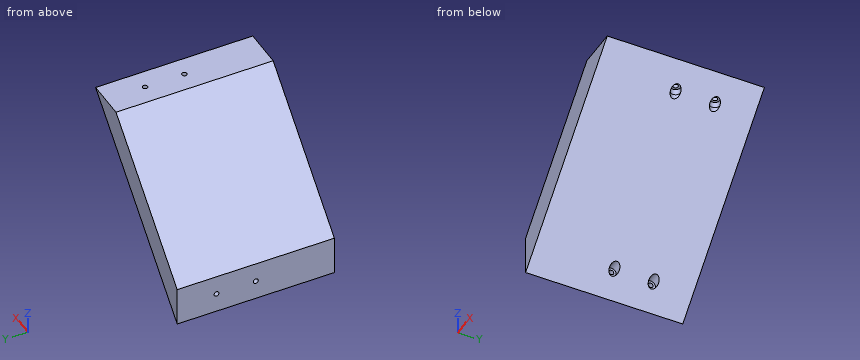
Autodesk Inventor part; units mm, degrees
ref_plane "YZ Plane" through (0, 0, 0) normal (1, 0, 0) x (0, 1, 0)
ref_plane "XZ Plane" through (0, 0, 0) normal (0, 1, 0) x (-1, 0, 0)
ref_plane "XY Plane" through (0, 0, 0) normal (0, 0, 1) x (1, 0, 0)
sketch "Sketch1" plane through (0, 0, 0) normal (0, 1, 0) x (-1, 0, 0)
  line L0 (6.35, 0) -> (1365.25, 0)
  line L1 (1371.6, -6.35) -> (1371.6, -1365.25)
  line L2 (1365.25, -1371.6) -> (6.35, -1371.6)
  line L3 (0, -1365.25) -> (0, -6.35)
  line L4 (1346.2, -1346.2) -> (1346.2, -25.4)
  line L5 (1346.2, -25.4) -> (25.4, -25.4)
  line L6 (25.4, -25.4) -> (25.4, -1346.2)
  line L7 (25.4, -1346.2) -> (1346.2, -1346.2)
  line L8 (1320.8, -50.8) -> (1320.8, -1320.8)
  line L9 (1320.8, -1320.8) -> (50.8, -1320.8)
  line L10 (50.8, -1320.8) -> (50.8, -50.8)
  line L11 (50.8, -50.8) -> (1320.8, -50.8)
  line L12 (1320.8, -50.8) -> (1346.2, -25.4)
  line L13 (1320.8, -1320.8) -> (1346.2, -1346.2)
  line L14 (50.8, -1320.8) -> (25.4, -1346.2)
  line L15 (50.8, -50.8) -> (25.4, -25.4)
  line L16 (1219.2, -482.6) -> (1016, -482.6)
  line L17 (1016, -482.6) -> (1016, -889)
  line L18 (1016, -889) -> (1219.2, -889)
  line L19 (1219.2, -889) -> (1219.2, -482.6)
  line L20 (355.6, -482.6) -> (152.4, -482.6)
  line L21 (152.4, -482.6) -> (152.4, -889)
  line L22 (152.4, -889) -> (355.6, -889)
  line L23 (355.6, -889) -> (355.6, -482.6)
  line L24 (889, -1016) -> (482.6, -1016)
  line L25 (482.6, -1016) -> (482.6, -1219.2)
  line L26 (482.6, -1219.2) -> (889, -1219.2)
  line L27 (889, -1219.2) -> (889, -1016)
  line L28 (889, -152.4) -> (482.6, -152.4)
  line L29 (482.6, -152.4) -> (482.6, -355.6)
  line L30 (482.6, -355.6) -> (889, -355.6)
  line L31 (889, -355.6) -> (889, -152.4)
  circle A0 centre (685.8, -685.8) radius 254
  line L32 (889, -127) -> (482.6, -127)
  line L33 (457.2, -127) -> (457.2, -381)
  line L34 (457.2, -381) -> (914.4, -381)
  line L35 (914.4, -381) -> (914.4, -127)
  line L36 (1244.6, -457.2) -> (990.6, -457.2)
  line L37 (990.6, -457.2) -> (990.6, -914.4)
  line L38 (990.6, -914.4) -> (1244.6, -914.4)
  line L39 (1244.6, -889) -> (1244.6, -482.6)
  line L40 (914.4, -990.6) -> (457.2, -990.6)
  line L41 (457.2, -990.6) -> (457.2, -1244.6)
  line L42 (482.6, -1244.6) -> (889, -1244.6)
  line L43 (914.4, -1244.6) -> (914.4, -990.6)
  line L44 (381, -457.2) -> (127, -457.2)
  line L45 (127, -482.6) -> (127, -889)
  line L46 (127, -914.4) -> (381, -914.4)
  line L47 (381, -914.4) -> (381, -457.2)
  line L48 (152.4, -482.6) -> (50.8, -482.6)
  line L49 (127, -457.2) -> (50.8, -457.2)
  line L50 (152.4, -889) -> (50.8, -889)
  line L51 (127, -914.4) -> (50.8, -914.4)
  line L52 (355.6, -889) -> (381, -889)
  line L53 (355.6, -482.6) -> (381, -482.6)
  line L54 (457.2, -1244.6) -> (457.2, -1320.8)
  line L55 (482.6, -1219.2) -> (482.6, -1320.8)
  line L56 (889, -1219.2) -> (889, -1320.8)
  line L57 (914.4, -1244.6) -> (914.4, -1320.8)
  line L58 (1244.6, -914.4) -> (1320.8, -914.4)
  line L59 (1219.2, -889) -> (1320.8, -889)
  line L60 (1219.2, -482.6) -> (1320.8, -482.6)
  line L61 (1244.6, -457.2) -> (1320.8, -457.2)
  line L62 (889, -152.4) -> (889, -50.8)
  line L63 (914.4, -127) -> (914.4, -50.8)
  line L64 (482.6, -152.4) -> (482.6, -50.8)
  line L65 (457.2, -127) -> (457.2, -50.8)
  line L66 (889, -1016) -> (889, -990.6)
  line L67 (482.6, -1016) -> (482.6, -990.6)
  line L68 (1016, -889) -> (990.6, -889)
  line L69 (1016, -482.6) -> (990.6, -482.6)
  line L70 (889, -355.6) -> (889, -381)
  line L71 (482.6, -355.6) -> (482.6, -381)
  line L72 (914.4, -381) -> (990.6, -457.2)
  line L73 (990.6, -482.6) -> (889, -381)
  line L74 (990.6, -914.4) -> (914.4, -990.6)
  line L75 (889, -990.6) -> (990.6, -889)
  line L76 (381, -914.4) -> (457.2, -990.6)
  line L77 (482.6, -990.6) -> (381, -889)
  line L78 (457.2, -381) -> (381, -457.2)
  line L79 (482.6, -381) -> (381, -482.6)
  line L80 (1257.3, -50.8) -> (1320.8, -114.3)
  line L81 (1320.8, -1257.3) -> (1257.3, -1320.8)
  line L82 (50.8, -1257.3) -> (114.3, -1320.8)
  line L83 (50.8, -114.3) -> (114.3, -50.8)
  line L84 (68.7605, -132.2605) -> (132.2605, -68.7605)
  line L85 (68.7605, -1239.3395) -> (132.2605, -1302.8395)
  line L86 (1302.8395, -1239.3395) -> (1239.3395, -1302.8395)
  line L87 (1239.3395, -68.7605) -> (1302.8395, -132.2605)
  line L88 (1302.8395, -132.2605) -> (1320.8, -150.221)
  line L89 (1239.3395, -68.7605) -> (1221.379, -50.8)
  line L90 (1302.8395, -1239.3395) -> (1320.8, -1221.379)
  line L91 (1239.3395, -1302.8395) -> (1221.379, -1320.8)
  line L92 (132.2605, -1302.8395) -> (150.221, -1320.8)
  line L93 (68.7605, -1239.3395) -> (50.8, -1221.379)
  line L94 (132.2605, -68.7605) -> (150.221, -50.8)
  line L95 (68.7605, -132.2605) -> (50.8, -150.221)
  line L96 (1365.25, 0) -> (1371.6, -6.35)
  line L97 (1371.6, -1365.25) -> (1365.25, -1371.6)
  line L98 (6.35, -1371.6) -> (0, -1365.25)
  line L99 (6.35, 0) -> (0, -6.35)
  point P0 (0, 0)
  point P1 (1371.6, -1371.6)
  point P2 (1371.6, 0)
  point P3 (0, -1371.6)
  dimension "d0" = 1371.6
  dimension "d1" = 1371.6
  dimension "d2" = 25.4
  dimension "d3" = 25.4
  dimension "d4" = 203.2
  dimension "d5" = 406.4
  dimension "d6" = 203.2
  dimension "d7" = 406.4
  dimension "d8" = 406.4
  dimension "d9" = 203.2
  dimension "d10" = 406.4
  dimension "d11" = 203.2
  dimension "d12" = 101.6
  dimension "d13" = 101.6
  dimension "d14" = 101.6
  dimension "d15" = 101.6
  dimension "d16" = 431.8
  dimension "d17" = 431.8
  dimension "d18" = 431.8
  dimension "d19" = 431.8
  dimension "d20" = 508
  dimension "d21" = 25.4
  dimension "d22" = 25.4
  dimension "d23" = 25.4
  dimension "d24" = 25.4
  dimension "d25" = 45
  dimension "d26" = 63.5
  dimension "d27" = 45
  dimension "d28" = 45
  dimension "d29" = 45
  dimension "d30" = 25.4
  dimension "d31" = 25.4
  dimension "d32" = 25.4
  dimension "d33" = 25.4
  dimension "d34" = 6.35
  dimension "d35" = 6.35
  dimension "d36" = 6.35
  dimension "d37" = 6.35
  dimension "d38" = 6.35
  dimension "d39" = 6.35
  dimension "d40" = 6.35
  dimension "d41" = 6.35
extrude "Extrusion1" add sketch "Sketch1" along normal blind 76.2 contours L37 L73 L34 L72
sketch "Sketch2" plane through (-914.4, 0, -381) normal (0, 0, 1) x (1, 0, 0)
  circle A0 centre (12.7, 50.8) radius 1.5875
  circle A1 centre (12.7, 25.4) radius 1.5875
  line L0 (25.4, 0) -> (25.4, 76.2)
  line L1 (0, 76.2) -> (25.4, 76.2)
  line L2 (0, 0) -> (25.4, 0)
  point P0 (914.4, 0)
  point P1 (12.7, 76.2)
  dimension "d44" = 3.175
  dimension "d45" = 3.175
  dimension "d46" = 12.7
  dimension "d47" = 25.4
  dimension "d48" = 25.4
  dimension "d49" = 12.7
extrude "Extrusion2" cut sketch "Sketch2" against normal blind 76.2
sketch "Sketch3" plane through (-990.6, 0, -482.6) normal (-1, 0, 0) x (0, 0, 1)
  circle A0 centre (12.7, 25.4) radius 1.5875
  circle A1 centre (12.7, 50.8) radius 1.5875
  line L0 (0, 0) -> (0, 76.2)
  line L1 (0, 76.2) -> (25.4, 76.2)
  line L2 (0, 0) -> (25.4, 0)
  point P0 (482.6, 0)
  point P1 (12.7, 76.2)
  dimension "d52" = 3.175
  dimension "d53" = 3.175
  dimension "d54" = 12.7
  dimension "d55" = 12.7
  dimension "d56" = 25.4
  dimension "d57" = 25.4
extrude "Extrusion3" cut sketch "Sketch3" against normal blind 76.2
hole "Hole1" at (-977.9, 50.8, -469.9) direction (1, 0, 0) diameter 6.35 depth 3.81
hole "Hole2" at (-977.9, 25.4, -469.9) direction (1, 0, 0) diameter 6.35 depth 3.81
hole "Hole3" at (-901.7, 50.8, -393.7) direction (0, 0, -1) diameter 6.35 depth 3.81
hole "Hole4" at (-901.7, 25.4, -393.7) direction (0, 0, -1) diameter 6.35 depth 3.81
hole "Hole5" at (-977.9, 50.8, -469.9) direction (-1, 0, 0) diameter 6.35 depth 3.81
hole "Hole6" at (-977.9, 25.4, -469.9) direction (-1, 0, 0) diameter 6.35 depth 3.81
hole "Hole7" at (-901.7, 25.4, -393.7) direction (0, 0, 1) diameter 6.35 depth 3.81
hole "Hole8" at (-901.7, 50.8, -393.7) direction (0, 0, 1) diameter 6.35 depth 3.81
sketch "Sketch4" plane through (0, 76.2, 0) normal (0, 1, 0) x (1, 0, 0)
  point P0 (0, 0)
sketch "Sketch5" plane through (0, 0, 0) normal (0, -1, 0) x (1, 0, 0)
  line L0 (-914.4, -381) -> (-889, -381)
  line L1 (-990.6, -457.2) -> (-914.4, -381)
  line L2 (-990.6, -482.6) -> (-990.6, -457.2)
  line L3 (-889, -381) -> (-990.6, -482.6)
  point P0 (0, 0)
extrude "Extrusion4" add sketch "Sketch5" along normal blind 25.4
properties part number "angle interior piece X4"
Geometry: final body of the model. Coordinates: model frame, mm. Give positions to 0.01 mm unless a question says otherwise; leave off trailing zeros. Write each loop counter-clockwise with the first axis right and the second up, starting at its lowest first coordinate (ties: lowest second). Pieces come first, ordered by that corner, then holes. Notation, with made-up numbers: (60, 18.5) -> (112, 18.5) arc R15 ccw to (112, 47.5) -> close; hole circle Ø11 at (-3.75, 58). An arc over 180 degrees is marked (long way). Answer as a JSON object with one key per item and string values.
1. Cut plane D-D on x = -919. Output: boundary loops of the cut face in (y, z), and give its area (3 significant figures).
Ans:
{"outline": "(-25.4, -411) -> (76.2, -411) -> (76.2, -385.6) -> (-25.4, -385.6) -> close", "area": "2,580 mm^2"}
2. Ray query, probe 1 along Y at (x, z) = (-988.5, -469.9); probe 2 along Y at (x, z) = (-901, -392); probe 3 along X at (y, z) = (10.5, -416). Return the intervals inside material, ascending. Write a range as from..to.
Ans:
{"probe 1": "y = -25.4..23.81, 26.99..49.21, 52.39..76.2", "probe 2": "y = -25.4..22.3, 28.5..47.7, 53.9..76.2", "probe 3": "x = -949.4..-924"}
3. Cut plane A-A on z = -469.9. Output: boundary loops of the cut face in (x, y) (1 decimal), and give its area (3 significant figures).
Ans:
{"outline": "(-990.6, -25.4) -> (-977.9, -25.4) -> (-977.9, 22.2) -> (-981.7, 22.2) -> (-981.7, 23.8) -> (-990.6, 23.8) -> close; (-990.6, 27) -> (-981.7, 27) -> (-981.7, 28.6) -> (-977.9, 28.6) -> (-977.9, 47.6) -> (-981.7, 47.6) -> (-981.7, 49.2) -> (-990.6, 49.2) -> close; (-990.6, 52.4) -> (-981.7, 52.4) -> (-981.7, 54) -> (-977.9, 54) -> (-977.9, 76.2) -> (-990.6, 76.2) -> close", "area": "1,190 mm^2"}
4. Contact query for flat-ended pins moving along their axis: pin 1 (4 mm diameter, centred on y = 32.5, z = -395, fed in from -X); pin 2 (3.5 mm diameter, centred on y = 25.4, z = -469.9, fed in from -X); pin 3 (7 mm diameter, centred on x = -902.5, y = 27, fed in from -Z); pin 4 (1.5 mm diameter, centred on y = 32, z = -402.5, fed in from -X). Output: stop coordinate, or through.
Ans:
{"pin 1": "stops at x = -930.4", "pin 2": "stops at x = -990.6", "pin 3": "stops at z = -398", "pin 4": "stops at x = -936.65"}
5. Cut plane B-B on y = 25.4. Output: boundary loops of the cut face in (x, z) (1 decimal).
Ans:
{"outline": "(-990.6, -482.6) -> (-981.1, -473.1) -> (-981.7, -473.1) -> (-981.7, -471.5) -> (-990.6, -471.5) -> close; (-990.6, -468.3) -> (-981.7, -468.3) -> (-981.7, -466.7) -> (-974.7, -466.7) -> (-904.9, -396.9) -> (-904.9, -389.9) -> (-903.3, -389.9) -> (-903.3, -381) -> (-914.4, -381) -> (-990.6, -457.2) -> close; (-900.1, -389.9) -> (-898.5, -389.9) -> (-898.5, -390.5) -> (-889, -381) -> (-900.1, -381) -> close"}
6. Cut plane C-C on z = -398.5. Output: boundary loops of the cut face in (x, y), and give its area (3 significant figures).
Ans:
{"outline": "(-931.9, -25.4) -> (-906.5, -25.4) -> (-906.5, 76.2) -> (-931.9, 76.2) -> close", "area": "2,580 mm^2"}
